Read the model definition and answer for the solid it produces. Units are mm, in the model's axes. Face numbers are marked on the shaded views. A direction names the side the tool comes from. Coordinates: 2 decimals unless noted, no trailing zeros. Write each loop counter-clockwise with the first axis right and the second up, starting at its lowest first coordinate (ties: lowest second). Pieces come first, ordered by that corner, then holes.
1) Find the intervals of material crossed by line 1 (X direction, y = 17.5, z = -2); line 2 (Y direction, x = -27.5, z = 1); line 3 (Y direction, x = -35, z = -4), in increasing order.
2) Each of these flat-tipped pins is pushed along its axis until it touches: pin 1 Ø1 at (x, y) = (-14, 16.5) entering from -Z; pin 2 Ø1 at (x, z) = (34.5, 0) entering from +Y; pin 3 Ø3 at (y, z) = (15.5, 0) entering from +X. Where does it stop, or does it pass through?
3) The part is cut by section D-D (y = 17.5). Determine the outline of the cut face in (x, z), then the cut area to 3 significant figures.
4) The part is cut by section A-A (z = 0). Determine the outline of the cut face in (x, y).
5) The part is cut by section B-B (y = 12.5). Determine the outline of the cut face in (x, z), then the cut area to 3 significant figures.
6) The part is cut by section C-C (x = 6). Determine the outline of the cut face in (y, z).
7) Which of the six approach directions +Z, -Z, +X, -X, +Y, -Y give full straight-line access (tool end or side, diameter ignored) to the marked faces 1, 2 and 3?
from build123d import *

# Parameters (mm, degrees)
SKETCH1_W           = 100
SKETCH1_H           = 5
SKETCH4_W           = 2
SKETCH4_H           = 9.797958971
BOSS_EXTRUDE4_DEPTH = 20
CUT_EXTRUDE5_DEPTH  = 2
SKETCH11_R          = 2.5
CUT_EXTRUDE6_DEPTH  = 2


with BuildPart() as part:
    # Sketch1 → Revolve1 (revolve)
    with BuildSketch(Plane.XY):
        with Locations((-23.848684211, 16.332236842)):
            Rectangle(SKETCH1_W, SKETCH1_H)
    revolve(axis=Axis((-73.848684211, 13.832236842, 0), (1, 0, 0)))

    # Sketch4 → Boss-Extrude4 (add)
    with BuildSketch(Plane(origin=(26.151315789, 0, 0), x_dir=(0, 0, -1), z_dir=(1, 0, 0))):
        with Locations((0, 13.832236843)):
            Rectangle(SKETCH4_W, SKETCH4_H)
    extrude(amount=BOSS_EXTRUDE4_DEPTH)

    # Sketch10 → Cut-Extrude5 (cut)
    with BuildSketch(Plane.XY.offset(1)):
        with BuildLine():
            Line((37.327139049, 18.731216328), (46.151315789, 18.731216328))
            Line((46.151315789, 18.731216328), (46.151315789, 8.933257357))
            Line((46.151315789, 8.933257357), (37.327139049, 8.933257357))
            ThreePointArc((37.327139049, 8.933257357), (42.226118535, 13.832236842), (37.327139049, 18.731216328))
        make_face()
    extrude(amount=-CUT_EXTRUDE5_DEPTH, mode=Mode.SUBTRACT)

    # Sketch11 → Cut-Extrude6 (cut)
    with BuildSketch(Plane.XY.offset(1)):
        with Locations((37.327139049, 13.832236842)):
            Circle(SKETCH11_R)
    extrude(amount=-CUT_EXTRUDE6_DEPTH, mode=Mode.SUBTRACT)


solid = part.part
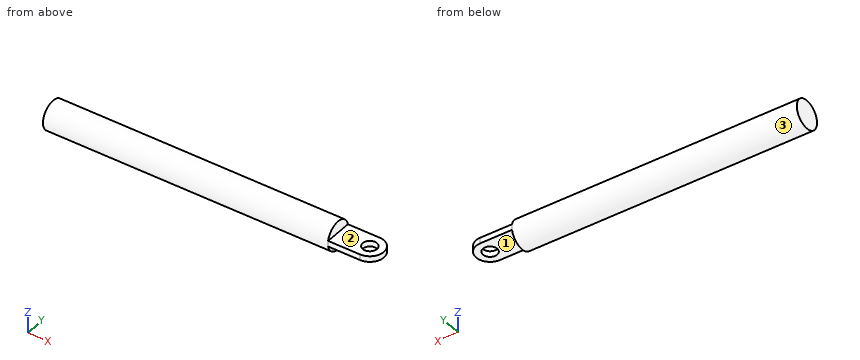
Reported:
1. line 1: x = -73.85 to 26.15
1. line 2: y = 8.93 to 18.73
1. line 3: y = 10.83 to 16.83
2. pin 1: stops at z = -4.51
2. pin 2: stops at y = 18.73
2. pin 3: stops at x = 42.22
3. outline: (-73.85, -3.4) - (26.15, -3.4) - (26.15, -1) - (40.57, -1) - (40.57, 1) - (26.15, 1) - (26.15, 3.4) - (-73.85, 3.4) - close
3. area: 708 mm2
4. outline: (-73.85, 8.83) - (26.15, 8.83) - (26.15, 8.93) - (37.33, 8.93) arc R4.9 ccw to (37.33, 18.73) - (26.15, 18.73) - (26.15, 18.83) - (-73.85, 18.83) - close; hole circle Ø5 at (37.33, 13.83)
5. outline: (-73.85, -4.82) - (26.15, -4.82) - (26.15, -1) - (35.21, -1) - (35.21, 1) - (26.15, 1) - (26.15, 4.82) - (-73.85, 4.82) - close; (39.44, -1) - (42.04, -1) - (42.04, 1) - (39.44, 1) - close
5. area: 987 mm2
6. outline: circle Ø10 at (13.83, 0)
7. face 1: -Z, +X, +Y, -Y
7. face 2: +Z, +X, +Y, -Y
7. face 3: +X, -X
